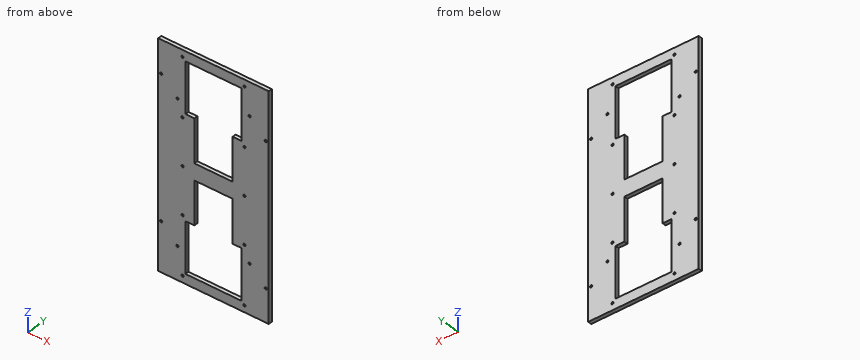
Autodesk Inventor part; units mm, degrees
ref_plane "YZ Plane" through (0, 0, 0) normal (1, 0, 0) x (0, 1, 0)
ref_plane "XZ Plane" through (0, 0, 0) normal (0, 1, 0) x (-1, 0, 0)
ref_plane "XY Plane" through (0, 0, 0) normal (0, 0, 1) x (1, 0, 0)
sketch "Esquisse1" plane through (0, 0, 0) normal (0, 1, 0) x (-1, 0, 0)
  line L0 (81.9588, 98.0854) -> (-68.0412, 98.0854)
  line L1 (-68.0412, 98.0854) -> (-68.0412, -201.9146)
  line L2 (-68.0412, -201.9146) -> (81.9588, -201.9146)
  line L3 (81.9588, -201.9146) -> (81.9588, 98.0854)
  point P0 (0, 0)
  dimension "d0" = 300
  dimension "d1" = 150
extrude "Extrusion1" add sketch "Esquisse1" along normal blind 5
sketch "Sketch3" plane through (0, 5, 0) normal (0, 1, 0) x (1, 0, 0)
  line L0 (31.0412, -85.0854) -> (-44.9588, -85.0854)
  line L1 (-44.9588, -85.0854) -> (-44.9588, -17.0854)
  line L2 (31.0412, -17.0854) -> (31.0412, -85.0854)
  line L3 (-81.9588, -98.0854) -> (68.0412, -98.0854)
  line L4 (68.0412, -98.0854) -> (68.0412, 201.9146)
  line L5 (-32.9588, -17.0854) -> (-32.9588, 40.9146)
  line L6 (-32.9588, 40.9146) -> (19.0412, 40.9146)
  line L7 (19.0412, 40.9146) -> (19.0412, -17.0854)
  line L8 (-44.9588, -17.0854) -> (-32.9588, -17.0854)
  line L9 (19.0412, -17.0854) -> (31.0412, -17.0854)
  line L10 (31.0412, 188.9146) -> (-44.9588, 188.9146)
  line L11 (-44.9588, 188.9146) -> (-44.9588, 120.9146)
  line L12 (31.0412, 120.9146) -> (31.0412, 188.9146)
  line L13 (68.0412, 201.9146) -> (-81.9588, 201.9146)
  line L14 (-32.9588, 120.9146) -> (-32.9588, 62.9146)
  line L15 (-32.9588, 62.9146) -> (19.0412, 62.9146)
  line L16 (19.0412, 62.9146) -> (19.0412, 120.9146)
  line L17 (-44.9588, 120.9146) -> (-32.9588, 120.9146)
  line L18 (19.0412, 120.9146) -> (31.0412, 120.9146)
  circle A0 centre (35.0412, 51.9146) radius 1.5
  line L19 (-81.9588, 201.9146) -> (-81.9588, -98.0854)
  circle A1 centre (-48.9588, 51.9146) radius 1.5
  point P0 (0, 0)
  dimension "d17" = 76
  dimension "d18" = 68
  dimension "d19" = 13
  dimension "d20" = 37
  dimension "d21" = 12
  dimension "d22" = 12
  dimension "d23" = 58
  dimension "d24" = 68
  dimension "d25" = 52
  dimension "d26" = 13
  dimension "d27" = 76
  dimension "d28" = 68
  dimension "d29" = 37
  dimension "d30" = 12
  dimension "d31" = 12
  dimension "d32" = 58
  dimension "d33" = 52
  dimension "d34" = 68
  dimension "d39" = 3
  dimension "d53" = 33
  dimension "d54" = 150
  dimension "d58" = 3
  dimension "d59" = 33
  dimension "d60" = 150
extrude "Extrusion3" cut sketch "Sketch3" against normal through all contours L0 L1 L8 L5 L6 L7 L9 L2 | L12 L18 L16 L15 L14 L17 L11 L10 | A0 | A1
sketch "Esquisse10" plane through (0, 5, 0) normal (0, 1, 0) x (1, 0, 0)
  circle A0 centre (-48.9588, -89.0854) radius 1.5
  circle A1 centre (-48.9588, -11.0854) radius 1.5
  circle A2 centre (-48.9588, 114.9146) radius 1.5
  circle A3 centre (-48.9588, 192.9146) radius 1.5
  circle A4 centre (35.0412, 192.9146) radius 1.5
  circle A5 centre (35.0412, 114.9146) radius 1.5
  circle A6 centre (35.0412, -11.0854) radius 1.5
  circle A7 centre (35.0412, -89.0854) radius 1.5
  point P0 (0, 0)
extrude "Extrusion9" cut sketch "Esquisse10" against normal through all
sketch "Esquisse12" plane through (0, 0, 0) normal (0, -1, 0) x (1, 0, 0)
  circle A0 centre (-77.9588, 54.0854) radius 1.5
  circle A1 centre (-55.9588, 32.0854) radius 1.5
  circle A2 centre (42.0412, 54.0854) radius 1.5
  circle A3 centre (64.0412, 32.0854) radius 1.5
  circle A4 centre (42.0412, -135.9146) radius 1.5
  circle A5 centre (64.0412, -157.9146) radius 1.5
  circle A6 centre (-55.9588, -157.9146) radius 1.5
  circle A7 centre (-77.9588, -135.9146) radius 1.5
  point P0 (0, 0)
extrude "Extrusion10" cut sketch "Esquisse12" against normal through all
properties part number "socle-robot"
Verification items for the finished model (mm, model axes). Coordinates: 2 decimals unless noted, no trailing zeros. Loops run counter-clockwise (first coordinate to the right, second up) from the corner with the lowest first, then second, coordinate; pieces in that order, holes last. Notation, with made-up numbers: (50, 61) -> (72, 61) arc R21 cw to (72, 74) -> close; hole circle Ø1 at (15, -33). An arc over 180 degrees is marked (long way). Write each question's results on one line, items separated by ' | '.
Item 1: Section check C-C, the plane z = 70.5. Enter the section's corners in (x, y).
Found:
outline: (-81.96, 0) -> (-44.96, 0) -> (-44.96, 5) -> (-81.96, 5) -> close; (31.04, 0) -> (68.04, 0) -> (68.04, 5) -> (31.04, 5) -> close
Item 2: Material ranges on L1, parallel to Z at x = -11.5, y = 4.4; L2, parallel to X at y = 4.55, z = 67; L3, parallel to X at y = 3.75, z = -34, recorded low to high.
Found:
L1: z = -201.91 to -188.91, -62.91 to -40.91, 85.09 to 98.09 | L2: x = -81.96 to -44.96, 31.04 to 68.04 | L3: x = -81.96 to -32.96, 19.04 to 68.04
Item 3: Section check D-D, the plane y = 1.5. Count the separate pieces of the cut face and the enclosed holes in it, plus the area to 3 significant figures.
Found:
separate pieces: 1 | enclosed holes: 20 | area: 28,500 mm2
Item 4: Section check B-B, the plane x = -17. Enter the section's corners in (y, z), plus the area to 3 significant figures.
Found:
outline: (0, -201.91) -> (5, -201.91) -> (5, -188.91) -> (0, -188.91) -> close; (0, -62.91) -> (5, -62.91) -> (5, -40.91) -> (0, -40.91) -> close; (0, 85.09) -> (5, 85.09) -> (5, 98.09) -> (0, 98.09) -> close | area: 240 mm2
Item 5: Section check A-A, the plane z = -82. Enter the section's corners in (x, y).
Found:
outline: (-81.96, 0) -> (-32.96, 0) -> (-32.96, 5) -> (-81.96, 5) -> close; (19.04, 0) -> (68.04, 0) -> (68.04, 5) -> (19.04, 5) -> close
